For this review, take the finished solid that the model builds, in its own axes (mm). A direction names the side the tool comes from. Coordinates: 2 decimals unless noted, no trailing zeros. Loops run counter-clockwise (first coordinate to the right, second up) from the corner with the lowest first, then second, coordinate; pieces in that order, holes last. Notation, with made-up numbers: M 0.25,61.5 L 54.25,61.5 A14 ccw 54.25,66.5 Z; hole C 18,-34.75 d11. An arc over 180 degrees is marked long. Put each result on its own line as item: value.
```python
from build123d import *

# Parameters (mm, degrees)
SKETCH_2_R                  = 8
EXTRUDE_2_DEPTH             = 190
EXTRUDE_3_DEPTH             = 190
SKETCH_7_R                  = 2.75
CUT_EXTRUDE_1_DEPTH         = 7
HOLE_WIZARD_M51_D           = 5.3
HOLE_WIZARD_M51_DEPTH       = 18
HOLE_WIZARD_M51_CBORE_D     = 10
HOLE_WIZARD_M51_CBORE_DEPTH = 5
HOLE_WIZARD_M51_TIP         = 1.59228064


with BuildPart() as part:
    # Эскиз2 → Бобышка-Вытянуть2 (new body)
    with BuildSketch(Plane.XY):
        Circle(SKETCH_2_R)
    extrude(amount=EXTRUDE_2_DEPTH)

    # Эскиз2<4> → Бобышка-Вытянуть3 (add)
    with BuildSketch(Plane.XY):
        with BuildLine():
            Line((9.355, -15.779924087), (4.181941588, -6.819924087))
            ThreePointArc((4.181941588, -6.819924087), (0, -8), (-4.181941588, -6.819924087))
            Line((-4.181941588, -6.819924087), (-9.355, -15.779924087))
            Line((-9.355, -15.779924087), (-25, -15.779924087))
            Line((-25, -15.779924087), (-25, -21.779924087))
            Line((-25, -21.779924087), (-9.355, -21.779924087))
            Line((-9.355, -21.779924087), (-8.748067357, -21.051410397))
            Line((-8.748067357, -21.051410397), (8.748067357, -21.051410397))
            Line((8.748067357, -21.051410397), (9.355, -21.779924087))
            Line((9.355, -21.779924087), (25, -21.779924087))
            Line((25, -21.779924087), (25, -15.779924087))
            Line((25, -15.779924087), (9.355, -15.779924087))
        make_face()
    extrude(amount=EXTRUDE_3_DEPTH)

    # Эскиз7 → Вырез-Вытянуть1 (cut, through all)
    with BuildSketch(Plane(origin=(0, -15.779924087, 0), x_dir=(1, 0, 0), z_dir=(0, 1, 0))):
        with Locations((-18.5, -170)):
            Circle(SKETCH_7_R)
        with Locations((18.5, -170)):
            Circle(SKETCH_7_R)
        with Locations((18.5, -20)):
            Circle(SKETCH_7_R)
        with Locations((-18.5, -20)):
            Circle(SKETCH_7_R)
    extrude(amount=-CUT_EXTRUDE_1_DEPTH, mode=Mode.SUBTRACT)

    # Цековка для винта с внутренним шестигранником M51
    with Locations(Plane(origin=(0, -21.051410397, 0), x_dir=(-1, 0, 0), z_dir=(0, -1, 0))):
        with Locations((0, -20), (0, -170)):
            CounterBoreHole(HOLE_WIZARD_M51_D / 2, HOLE_WIZARD_M51_CBORE_D / 2, HOLE_WIZARD_M51_CBORE_DEPTH, depth=HOLE_WIZARD_M51_DEPTH)
            with Locations((0, 0, -(HOLE_WIZARD_M51_DEPTH + HOLE_WIZARD_M51_TIP / 2))):  # 118° drill point
                Cone(0, HOLE_WIZARD_M51_D / 2, HOLE_WIZARD_M51_TIP, mode=Mode.SUBTRACT)


solid = part.part
```
(1) Tool access review of faces 4 (the cylindrical face through (0.651, -18.586, 165.043)), 5 (the flat face through (6.805, -11.363, 93.67)), 6 (the flat face through (17, -15.78, 94)): name each direction out of +Z, -Z, +X, -X, +Y, -Y from which nothing blocks a thin tool from reaching the whole face with its end or side.
Determined:
face 4: -Y
face 5: +Z, -Z, +X
face 6: +Z, -Z, +X, +Y
(2) Add section A-A (x = -18.5). Write out the cut boundary in (y, z), plus the area to 3 significant figures.
Determined:
outline: M -21.78,0 L -15.78,0 L -15.78,17.25 L -21.78,17.25 Z; M -21.78,22.75 L -15.78,22.75 L -15.78,167.25 L -21.78,167.25 Z; M -21.78,172.75 L -15.78,172.75 L -15.78,190 L -21.78,190 Z
area: 1,070 mm^2
(3) Add section D-D (y = -9). Write out the cut boundary in (x, z).
Determined:
outline: M -5.44,0 L 5.44,0 L 5.44,190 L -5.44,190 Z; hole C 0,20 d5.3; hole C 0,170 d5.3
(4) For pin 1 (6 mm diameter, centred on y = -7, z = 38.5, fed in from -X); pin 2 (7 mm diameter, centred on x = -18.5, z = 20, fed in from +Y); pin 3 (2 mm diameter, centred on y = 2.5, z = 68.5, fed in from -X); pin 4 (5 mm diameter, centred on x = -18.5, z = 170, fed in from -Y), all flat-tipped, find the tip position at first contact; note any pin that passes through.
Determined:
pin 1: stops at x = -6.93
pin 2: stops at y = -15.78
pin 3: stops at x = -7.86
pin 4: passes through
(5) Add section B-B (y = -19.25). Write out the cut boundary in (x, z).
Determined:
outline: M -25,0 L 25,0 L 25,190 L -25,190 Z; hole C -18.5,20 d5.5; hole C -18.5,170 d5.5; hole C 0,20 d10; hole C 0,170 d10; hole C 18.5,20 d5.5; hole C 18.5,170 d5.5
(6) Add section C-C (z = 155.5). Write out the cut boundary in (x, y) (3 decimals).
Determined:
outline: M -25,-21.78 L -9.355,-21.78 L -8.748,-21.051 L 8.748,-21.051 L 9.355,-21.78 L 25,-21.78 L 25,-15.78 L 9.355,-15.78 L 4.182,-6.82 A8 ccw long -4.182,-6.82 L -9.355,-15.78 L -25,-15.78 Z
(7) Wall thickness on line 1 along X through (y, z) = (-19.5, 20); line 2 along Z through (x, y) = (18.5, -18); line 3 along Z through (x, y) = (0, -17.45): over which ranges is each line inside the solid? List them lowest first. Write a range as [from, to].
Determined:
line 1: x = [-25, -21.25], [-15.75, -5], [5, 15.75], [21.25, 25]
line 2: z = [0, 17.25], [22.75, 167.25], [172.75, 190]
line 3: z = [0, 15], [25, 165], [175, 190]
(8) Draft analysis for pull direction Y (two halves, no side actions). For faces 1 (the conical face through (0.37, -1.74, 170.28)), 2 (the flat face through (0, -10, 190)), 3 (the cylindrical face through (0, 8, 94)), state which applies: +Y half, -Y half, draft (parallel to the pull), parting line (faces both ways), or undercut.
Determined:
face 1: -Y half
face 2: draft
face 3: undercut
